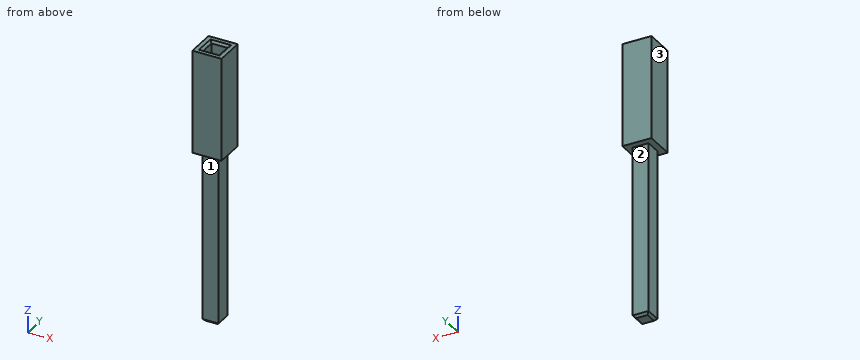
from build123d import *

# Parameters (mm, degrees)
F0_W     = 2.54
F0_H     = 2.54
F0_W_2   = 1.4
F0_H_2   = 1.4
F1_DEPTH = 9
F2_SIZE  = 0.2
F3_W     = 1.4
F3_H     = 1.4
F4_DEPTH = 15
F5_SIZE  = 0.2
F6_DEPTH = 0.5


with BuildPart() as f1:
    # F0 (on Top) → F1 (new body)
    with BuildSketch(Plane.XY):
        Rectangle(F0_W, F0_H)
        Rectangle(F0_W_2, F0_H_2, mode=Mode.SUBTRACT)
    extrude(amount=F1_DEPTH)

    # F2
    f2_edges = [f1.edges().sort_by_distance(p)[0] for p in [
        (0, -0.7, 9),
        (-0.7, 0, 9),
        (0, 0.7, 9),
        (0.7, 0, 9),
    ]]
    chamfer(f2_edges, length=F2_SIZE)

    # F3 (on face) → F4 (join)
    with BuildSketch(Plane(origin=(0, 0, 0), x_dir=(1, 0, 0), z_dir=(0, 0, -1))):
        Rectangle(F3_W, F3_H)
    extrude(amount=F4_DEPTH)

    # F5
    f5_edges = [f1.edges().sort_by_distance(p)[0] for p in [
        (-0.7, 0, -15),
        (0, 0.7, -15),
        (0.7, 0, -15),
        (0, -0.7, -15),
    ]]
    chamfer(f5_edges, length=F5_SIZE)

    # F6 (add): a face of the model
    f6_faces = [f1.faces().sort_by_distance(p)[0] for p in [
        (0, 0, 0),
    ]]
    extrude(f6_faces, amount=F6_DEPTH)


solid = f1.part
Could you check a few things on this model? Use its own coordinates, in mm. Face numbers are marked on the shaded views. A direction names the side the tool comes from. Give positions to 0.01 mm unless a question says otherwise; leave off trailing zeros. Order: outer loops, then holes, each group sorted by start corner. A loop starts at its lowest first (then second) coordinate and runs counter-clockwise, first axis right, second up.
Item 1: If we section it at D-D, the plane z = -9.25: Write out the boundary of the cut face in (x, y).
Item 2: For the marked faces 1, 2 and 3, which set-ups out of +Z, -Z, +X, -X, +Y, -Y let a thin tool reach every point of the face, with its end or its side?
Item 3: I'm going to push flat-ended pins straight in: pin 1 (1.1 mm diameter, centred on x = 0, z = -8.5, fed in from -Y); pin 2 (1.1 mm diameter, centred on y = 0, z = -11, fed in from -X); pin 3 (0.7 mm diameter, centred on y = 0, z = -11, fed in from +X); pin 4 (1.1 mm diameter, centred on x = -0.5, y = 0, fed in from +Z). Where does each tip first touch, or does it pass through?
Item 4: If we section it at A-A, the plane z = 0.75: Write out the boundary of the cut face in (x, y).
Item 5: I need wall thicknesses on line 1 (X direction, y = -0.15, z = 4.5); line 2 (Z direction, x = 0.95, y = -0.05); line 3 (Y direction, x = -0.65, z = -6). Which ranges of each line are inside material? Lowest first, please.
Item 6: If we section it at B-B, the plane x = 0.2: Write out the boundary of the cut face in (y, z), plus the area to 3 significant figures.
Values:
1. outline: (-0.7, -0.7) - (0.7, -0.7) - (0.7, 0.7) - (-0.7, 0.7) - close
2. face 1: -Z, +X, -X, -Y
2. face 2: -Z, +X, -X, +Y
2. face 3: +Z, -Z, -X, +Y, -Y
3. pin 1: stops at y = -0.7
3. pin 2: stops at x = -0.7
3. pin 3: stops at x = 0.7
3. pin 4: stops at z = 9
4. outline: (-1.27, -1.27) - (1.27, -1.27) - (1.27, 1.27) - (-1.27, 1.27) - close; hole (-0.7, -0.7) - (0.7, -0.7) - (0.7, 0.7) - (-0.7, 0.7) - close
5. line 1: x = -1.27 to -0.7, 0.7 to 1.27
5. line 2: z = 0 to 9
5. line 3: y = -0.7 to 0.7
6. outline: (-1.27, 0) - (-0.7, 0) - (-0.7, -14.8) - (-0.5, -15) - (0.5, -15) - (0.7, -14.8) - (0.7, 0) - (1.27, 0) - (1.27, 9) - (0.9, 9) - (0.7, 8.8) - (0.7, 0.5) - (-0.7, 0.5) - (-0.7, 8.8) - (-0.9, 9) - (-1.27, 9) - close
6. area: 31.9 mm2
